from build123d import *

# Parameters (mm, degrees)
F0_W      = 40
F0_H      = 60
F0_W_2    = 50
F0_W_3    = 3
F0_H_2    = 10
F1_DEPTH  = 3
F0_W_4    = 4
F0_H_3    = 30
F2_DEPTH  = 40
F3_DEPTH  = 12
F4_SIZE   = 1
F5_R      = 1.1
F6_DEPTH  = 13
F7_W      = 60
F7_H      = 60
F7_R      = 3
F7_R_2    = 4
F8_DEPTH  = 3
F10_DEPTH = 3
F12_DEPTH = 100
F14_DEPTH = 3
F15_SIZE  = 24.99999
F17_DEPTH = 30


# Not quite as in the source:
# - a fillet or chamfer is up to 0.001 mm smaller than in the source, because OpenCascade refuses the exact size
# - a feature names something its author has since deleted; it is built from what else it names


with BuildPart() as f1:
    # F0 (on Top) → F1 (new body)
    with BuildSketch(Plane.XY):
        with Locations((-20, -30)):
            Rectangle(F0_W, F0_H)
        with Locations((25, -30)):
            Rectangle(F0_W_2, F0_H)
        with Locations((14, -8)):
            Rectangle(F0_W_3, F0_H_2, mode=Mode.SUBTRACT)
        with Locations((23, -8)):
            Rectangle(F0_W_3, F0_H_2, mode=Mode.SUBTRACT)
        Polygon((0, 45), (0, 0), (50, 0), (50, 45), (41, 45), (41, 15), (37, 15), (37, 45), align=None)
        Polygon((-40, 0), (0, 0), (0, 45), (-26, 45), (-26, 15), (-30, 15), (-30, 45), (-40, 45), align=None)
    extrude(amount=F1_DEPTH)

    # F0 (on Top) → F2 (join)
    with BuildSketch(Plane.XY):
        with Locations((-28, 30)):
            Rectangle(F0_W_4, F0_H_3)
        with Locations((39, 30)):
            Rectangle(F0_W_4, F0_H_3)
    extrude(amount=F2_DEPTH)

    # F0 (on Top) → F3 (join)
    with BuildSketch(Plane.XY):
        with Locations((23, -8)):
            Rectangle(F0_W_3, F0_H_2)
        with Locations((14, -8)):
            Rectangle(F0_W_3, F0_H_2)
    extrude(amount=F3_DEPTH)

    # F4
    f4_edges = [f1.edges().sort_by_distance(p)[0] for p in [
        (14, -3, 12),
        (23, -3, 12),
        (23, -13, 12),
        (14, -13, 12),
    ]]
    chamfer(f4_edges, length=F4_SIZE)

    # F5 (on face) → F6 (cut)
    with BuildSketch(Plane.YZ.offset(24.5)):
        with Locations((-8, 8)):
            Circle(F5_R)
    extrude(amount=-F6_DEPTH, mode=Mode.SUBTRACT)

    # F7 (on Right) → F8 (join)
    with BuildSketch(Plane.YZ):
        with Locations((-30, 30)):
            Rectangle(F7_W, F7_H)
        with Locations((-45, 18)):
            Circle(F7_R, mode=Mode.SUBTRACT)
        with Locations((-14, 18)):
            Circle(F7_R, mode=Mode.SUBTRACT)
        with Locations((-45, 49)):
            Circle(F7_R, mode=Mode.SUBTRACT)
        with Locations((-29.5, 33.5)):
            Circle(F7_R_2, mode=Mode.SUBTRACT)
        with Locations((-14, 49)):
            Circle(F7_R, mode=Mode.SUBTRACT)
    extrude(amount=F8_DEPTH)

    # F9 (on Front) → F10 (join)
    with BuildSketch(Plane.XZ):
        Polygon((0, 60), (0, 0), (50, 0), (21.5, 34.2), (15.5, 41.4), (10, 48), (10, 43), (8, 43), (8, 50.4), align=None)
        Polygon((15.5, 41.4), (21.5, 34.2), (21.5, 49.2), (15.5, 49.2), align=None)
    extrude(amount=F10_DEPTH)

    # F11 (on face) → F12 (cut)
    with BuildSketch(Plane.YZ.offset(41)):
        with BuildLine():
            Line((21, 40), (23.2917960675, 40))
            ThreePointArc((23.2917960675, 40), (30, 43), (36.7082039325, 40))
            Line((36.7082039325, 40), (39, 40))
            Line((39, 40), (39, 47))
            Line((39, 47), (21, 47))
            Line((21, 47), (21, 40))
        make_face()
        with BuildLine():
            ThreePointArc((23.2917960675, 40), (21.5924487693, 37.211398808), (21, 34))
            ThreePointArc((21, 34), (30, 25), (39, 34))
            ThreePointArc((39, 34), (38.4075512307, 37.211398808), (36.7082039325, 40))
            Line((36.7082039325, 40), (23.2917960675, 40))
        make_face()
        with BuildLine():
            Line((21, 40), (21, 34))
            ThreePointArc((21, 34), (21.5924487693, 37.211398808), (23.2917960675, 40))
            Line((23.2917960675, 40), (21, 40))
        make_face()
        with BuildLine():
            ThreePointArc((36.7082039325, 40), (38.4075512307, 37.211398808), (39, 34))
            Line((39, 34), (39, 40))
            Line((39, 40), (36.7082039325, 40))
        make_face()
    extrude(amount=-F12_DEPTH, mode=Mode.SUBTRACT)

    # F13 (on face) → F14 (join)
    with BuildSketch(Plane.XZ.offset(60)):
        Polygon((3, 28), (3, 3), (28, 3), align=None)
    extrude(amount=-F14_DEPTH)

    # F15 (size 25 in the source; OpenCascade refuses exactly that, so slightly less here)
    f15_edges = [f1.edges().sort_by_distance(p)[0] for p in [
        (50, -60, 1.5),
        (-40, -60, 1.5),
    ]]
    chamfer(f15_edges, length=F15_SIZE)

    # F16 (on face) → F17 (join)
    with BuildSketch(Plane(origin=(0, 45, 0), x_dir=(-1, 0, 0), z_dir=(0, 1, 0))):
        Polygon((30, 3), (38, 3), (30, 18), align=None)
        Polygon((-49, 3), (-41, 3), (-41, 18), align=None)
    extrude(amount=-F17_DEPTH)


solid = f1.part
Model file for the job. Use its own axes, mm. A direction names the side the tool comes from. Coordinates: 2 decimals unless noted, no trailing zeros. Write each loop counter-clockwise with the first axis right and the second up, starting at its lowest first coordinate (ties: lowest second). Pieces come first, ordered by that corner, then holes. Notation, with made-up numbers: (-14, -20.5) - (29, -20.5) arc R26 cw to (29, 11.5) - close; hole circle Ø5 at (40, 77). An arc over 180 degrees is marked (long way). Write each question's results on one line, items separated by ' | '. Start each with the question number.
1) Cut at C-C (x = 43.5). Write the cut outline in (y, z), then the cut area to 3 significant figures.
2) Probe line 1 along Z through (x, y) = (1, -14); line 2 along X through (y, z) = (38, 18); line 3 along Z through (x, y) = (1.3, -29.5). List the from-to ranges inside material, lowest first. Write a range as from..to.
3) Flat gauge pins, fed straight in: P1, Ø2.5, axis at y = -6.5, z = 9, coming from the -X side; P2, Ø4.5, axis at x = 39, z = 38, coming from the -Y side; P3, Ø10, axis at x = 13.5, z = 11.5, coming from the +Y side. Where does each tip first touch, or does it go through?
4) Cut at A-A (y = 17). Write the cut outline in (x, z).
5) Cut at B-B (y = -45). Write the cut outline in (x, z).
6) Mould opens along X. For faces 1 (the face through (1.5, -16.4, 16.2)), 2 (the face through (0, -30, 26)), 3 (the face through (37, 30, 17)) say: pulls with the +X half, pulls with the -X half, needs draft (parallel to the pull), parting line crosses it, or undercut.
7) Cut at D-D (y = 30). Write the cut outline in (x, z).
8) 3-axis set-ups, long thin cutter, end or side, ignore diameter. For faces 4 (the face through (10, -57, 10)), 5 (the face through (-26, 30, 17)), 6 (the face through (21.5, -1, 42)), 7 (the face through (23, -8, 12)), 8 (the face through (-30, 30, 24)): which of +Z, -Z, +X, -X, +Y, -Y reach the whole face in a straight line?
Returned:
1) outline: (-41.5, 0) - (45, 0) - (45, 13.31) - (15, 13.31) - (15, 3) - (0, 3) - (0, 7.8) - (-3, 7.8) - (-3, 3) - (-41.5, 3) - close | area: 583 mm^2
2) line 1: 0..15, 21..46, 52..60 | line 2: -30..-26, 37..41 | line 3: 0..29.5, 37.5..60
3) P1: x = 0 | P2: y = 15 | P3: y = 0
4) outline: (-40, 0) - (50, 0) - (50, 3) - (49, 3) - (41, 18) - (41, 40) - (37, 40) - (37, 3) - (-26, 3) - (-26, 40) - (-30, 40) - (-30, 18) - (-38, 3) - (-40, 3) - close
5) outline: (-30, 0) - (40, 0) - (40, 3) - (3, 3) - (3, 15) - (0, 15) - (0, 3) - (-30, 3) - close; (0, 21) - (3, 21) - (3, 46) - (0, 46) - close; (0, 52) - (3, 52) - (3, 60) - (0, 60) - close
6) face 1: needs draft | face 2: pulls with the -X half | face 3: undercut
7) outline: (-40, 0) - (50, 0) - (50, 3) - (49, 3) - (41, 18) - (41, 25) - (37, 25) - (37, 3) - (-26, 3) - (-26, 25) - (-30, 25) - (-30, 18) - (-38, 3) - (-40, 3) - close
8) face 4: +Z, +X | face 5: +Z, +Y, -Y | face 6: +Z, +X, +Y, -Y | face 7: +Z, +X, -Y | face 8: +Z, -X, +Y, -Y
